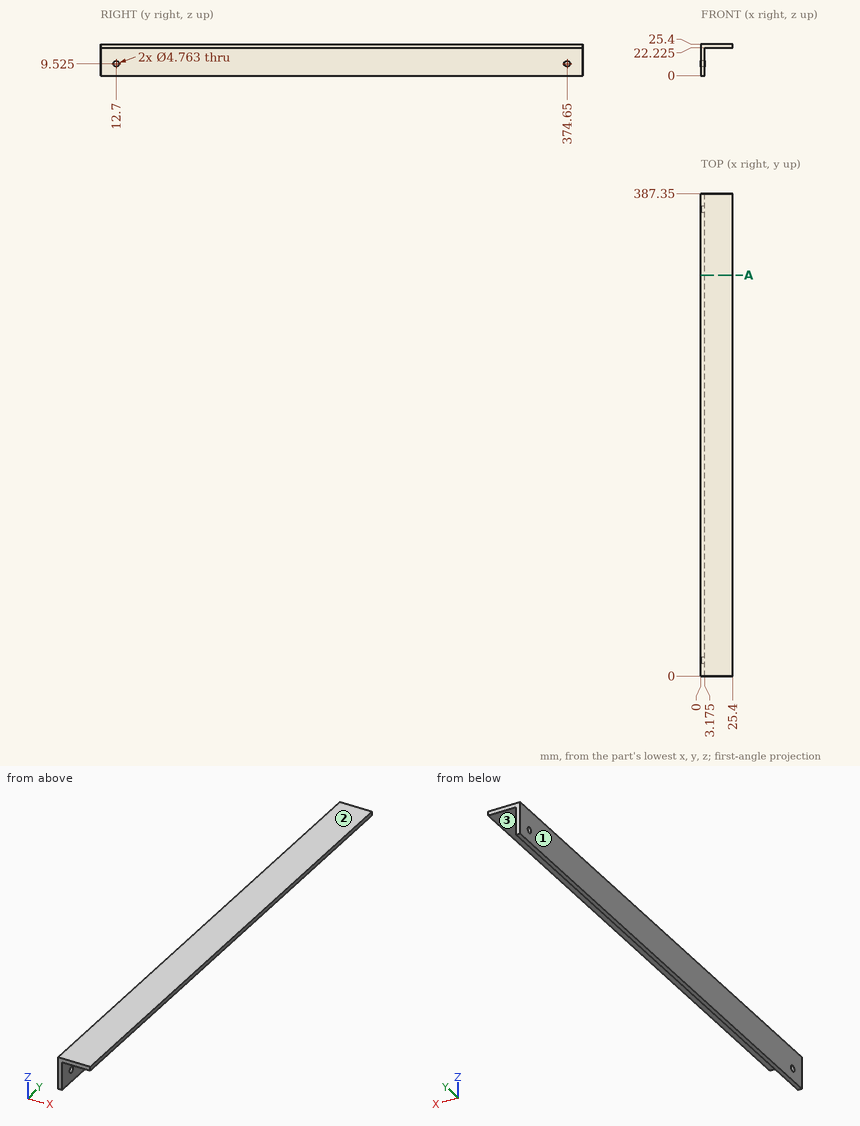
Here's the drawing with two shaded views (mm, measured from the low corner). I have some questions. Give positions to 0.01 mm unless a question says otherwise; leave off trailing zeros. Loops run counter-clockwise (first coordinate to the right, second up) from the corner with the lowest first, then second, coordinate; pieces in that order, holes last. Notation, with made-up numbers: M 19,71.25 L 59,71.25 A21 ccw 59,100.25 Z; hole C -3,50 d1. An arc over 180 degrees is marked long. One line per item, written item: value.
(1) Will these pins go through, and if not, where does the flat tip stop? pin 1 (5.5 mm diameter, centred on y = 374.65, z = 9.525, fed in from +X) (1 decimal); pin 2 (6 mm diameter, centred on x = 11, y = 90, fed in from -Z) (1 decimal); pin 3 (1.5 mm diameter, centred on y = 320.5, z = 20, fed in from -X).
Returned:
pin 1: x = 3.2
pin 2: z = 22.2
pin 3: x = 0
(2) Suppose I cut it at A-A on y = 322. List the corners of the cut face in (x, z) for me (1 decimal).
Returned:
outline: M 0,0 L 3.2,0 L 3.2,22.2 L 25.4,22.2 L 25.4,25.4 L 0,25.4 Z
(3) We'd pull the mould along Z, two halves only. Please class the marked faces 1, 2 and 3: released by +Z, released by -Z, zero draft, split by the parting line, or undercut.
Returned:
face 1: zero draft
face 2: released by +Z
face 3: released by -Z
(4) I need wall thicknesses on line 1 (Z direction, x = 1.25, y = 12.7); line 2 (Z direction, x = 8.75, y = 278) (1 decimal); line 3 (X direction, y = 247, z = 17.25) (1 decimal). Which ranges of each line are inside material? Lowest first, please.
Returned:
line 1: 0 to 7.14, 11.91 to 25.4
line 2: 22.2 to 25.4
line 3: 0 to 3.2
